The model under review builds one solid part; all positions refer to its coordinate system, in mm. Face numbers are marked on the shaded views. A direction names the side the tool comes from. Give positions to 0.01 mm unless a question says otherwise; leave off trailing zeros. Write each loop counter-clockwise with the first axis right and the second up, starting at its lowest first coordinate (ties: lowest second). Pieces come first, ordered by that corner, then holes.
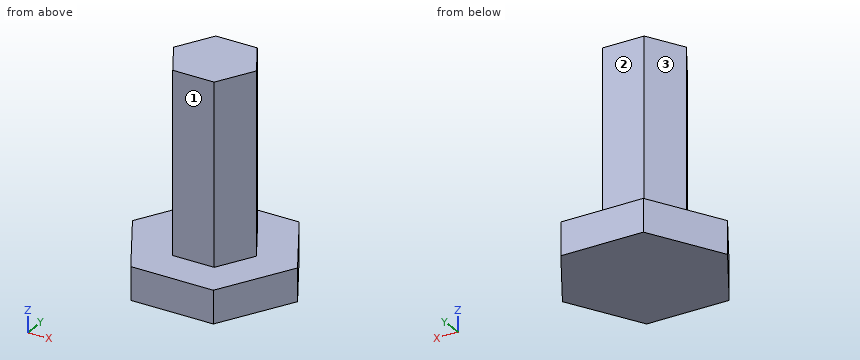
from build123d import *

# Parameters (mm, degrees)
BOSS_EXTRUDE1_DEPTH = 10
BOSS_EXTRUDE2_DEPTH = 2
MOVE_FACE1_BY       = 0.15
MOVE_FACE1_2_BY     = 0.15
MOVE_FACE1_3_BY     = 0.15
MOVE_FACE1_4_BY     = 0.15
MOVE_FACE1_5_BY     = 0.15
MOVE_FACE1_6_BY     = 0.15
MOVE_FACE1_7_BY     = 0.15
MOVE_FACE1_8_BY     = 0.15
MOVE_FACE1_9_BY     = 0.15
MOVE_FACE1_10_BY    = 0.15
MOVE_FACE1_11_BY    = 0.15
MOVE_FACE1_12_BY    = 0.15
MOVE_FACE1_13_BY    = 0.15


with BuildPart() as part:
    # Sketch1 → Boss-Extrude1 (new body)
    with BuildSketch(Plane.XY):
        Polygon((-2.5, 0), (-1.25, -2.165063509), (1.25, -2.165063509), (2.5, 0), (1.25, 2.165063509), (-1.25, 2.165063509), align=None)
    extrude(amount=BOSS_EXTRUDE1_DEPTH)

    # Sketch1_3 → Boss-Extrude2 (add)
    # profile 1 of 2: a face of its own
    with BuildSketch(Plane.XY):
        Polygon((-4.809401077, 0), (-2.404700538, -4.165063509), (2.404700538, -4.165063509), (4.809401077, 0), (2.404700538, 4.165063509), (-2.404700538, 4.165063509), align=None)
        Polygon((-1.25, -2.165063509), (1.25, -2.165063509), (2.5, 0), (1.25, 2.165063509), (-1.25, 2.165063509), (-2.5, 0), align=None, mode=Mode.SUBTRACT)
    # profile 2 of 2: a face of its own
    with BuildSketch(Plane.XY):
        Polygon((-2.5, 0), (-1.25, -2.165063509), (1.25, -2.165063509), (2.5, 0), (1.25, 2.165063509), (-1.25, 2.165063509), align=None)
    extrude(amount=-BOSS_EXTRUDE2_DEPTH)

    # Move Face1: a face moved inward by 0.15
    extrude(part.faces().sort_by_distance((0, -3.332050808, 0))[0], amount=MOVE_FACE1_BY, dir=(0, 0, -1), mode=Mode.SUBTRACT)

    # Move Face1 2: a face moved inward by 0.15
    extrude(part.faces().sort_by_distance((0, 4.165063509, -1))[0], amount=MOVE_FACE1_2_BY, dir=(0, -1, 0), mode=Mode.SUBTRACT)

    # Move Face1 3: a face moved inward by 0.15
    extrude(part.faces().sort_by_distance((3.607050808, 2.082531755, -1))[0], amount=MOVE_FACE1_3_BY, dir=(-0.866025404, -0.5, 0), mode=Mode.SUBTRACT)

    # Move Face1 4: a face moved inward by 0.15
    extrude(part.faces().sort_by_distance((3.607050808, -2.082531755, -1))[0], amount=MOVE_FACE1_4_BY, dir=(-0.866025404, 0.5, 0), mode=Mode.SUBTRACT)

    # Move Face1 5: a face moved inward by 0.15
    extrude(part.faces().sort_by_distance((0, -4.165063509, -1))[0], amount=MOVE_FACE1_5_BY, dir=(0, 1, 0), mode=Mode.SUBTRACT)

    # Move Face1 6: a face moved inward by 0.15
    extrude(part.faces().sort_by_distance((-3.607050808, 2.082531755, -1))[0], amount=MOVE_FACE1_6_BY, dir=(0.866025404, -0.5, 0), mode=Mode.SUBTRACT)

    # Move Face1 7: a face moved inward by 0.15
    extrude(part.faces().sort_by_distance((-3.607050808, -2.082531755, -1))[0], amount=MOVE_FACE1_7_BY, dir=(0.866025404, 0.5, 0), mode=Mode.SUBTRACT)

    # Move Face1 8: a face moved inward by 0.15
    extrude(part.faces().sort_by_distance((1.875, 1.082531755, 5))[0], amount=MOVE_FACE1_8_BY, dir=(-0.866025404, -0.5, 0), mode=Mode.SUBTRACT)

    # Move Face1 9: a face moved inward by 0.15
    extrude(part.faces().sort_by_distance((0, 2.165063509, 5))[0], amount=MOVE_FACE1_9_BY, dir=(0, -1, 0), mode=Mode.SUBTRACT)

    # Move Face1 10: a face moved inward by 0.15
    extrude(part.faces().sort_by_distance((-1.875, 1.082531755, 5))[0], amount=MOVE_FACE1_10_BY, dir=(0.866025404, -0.5, 0), mode=Mode.SUBTRACT)

    # Move Face1 11: a face moved inward by 0.15
    extrude(part.faces().sort_by_distance((-1.875, -1.082531755, 5))[0], amount=MOVE_FACE1_11_BY, dir=(0.866025404, 0.5, 0), mode=Mode.SUBTRACT)

    # Move Face1 12: a face moved inward by 0.15
    extrude(part.faces().sort_by_distance((0, -2.165063509, 5))[0], amount=MOVE_FACE1_12_BY, dir=(0, 1, 0), mode=Mode.SUBTRACT)

    # Move Face1 13: a face moved inward by 0.15
    extrude(part.faces().sort_by_distance((1.875, -1.082531755, 5))[0], amount=MOVE_FACE1_13_BY, dir=(-0.866025404, 0.5, 0), mode=Mode.SUBTRACT)


solid = part.part
1) Consider section D-D, the plane z = -1.25. Give the boundary of the cut face in (x, y), then the cut area to 3 significant figures.
2) Insertion check: pin 1 (0.7 mm diameter, centred on x = 0.5, z = 5.5, fed in from +Y); pin 2 (2 mm diameter, centred on y = -2.5, z = 5, fed in from +X); pin 3 (1.2 mm diameter, centred on x = 0, z = 3, fed in from -Y). Each pin has a flat end and moves straight along its axis. Give the tip position at first contact, or say it passes through.
3) Consider section B-B, the plane z = 1. Give the boundary of the cut face in (x, y).
4) To check wall thickness, follow probe 1 along Z at (x, y) = (-1.5, -1.75); probe 2 along Y at (x, z) = (0, 7.5); probe 3 along X at (y, z) = (1.75, 5.5). State the ranges of each line that lie inside material, in increasing order.
5) Consider section A-A, the plane x = 0.75. Give the boundary of the cut face in (y, z).
6) Tool access review of the marked faces 1, 2 and 3: name each direction out of +Z, -Z, +X, -X, +Y, -Y from which nothing blocks a thin tool from reaching the whole face with its end or side.
7) Consider section C-C, the plane y = -0.25. Give the boundary of the cut face in (x, z), then the cut area to 3 significant figures.
Answer block:
1. outline: (-4.64, 0) - (-2.32, -4.02) - (2.32, -4.02) - (4.64, 0) - (2.32, 4.02) - (-2.32, 4.02) - close
1. area: 55.8 mm2
2. pin 1: stops at y = 2.02
2. pin 2: stops at x = 1.46
2. pin 3: stops at y = -2.02
3. outline: (-2.33, 0) - (-1.16, -2.02) - (1.16, -2.02) - (2.33, 0) - (1.16, 2.02) - (-1.16, 2.02) - close
4. probe 1: z = -2 to -0.15
4. probe 2: y = -2.02 to 2.02
4. probe 3: x = -1.32 to 1.32
5. outline: (-4.02, -2) - (4.02, -2) - (4.02, -0.15) - (2.02, -0.15) - (2.02, 10) - (-2.02, 10) - (-2.02, -0.15) - (-4.02, -0.15) - close
6. face 1: +Z, +X, -X, -Y
6. face 2: +Z, +X, -X, +Y
6. face 3: +Z, -X, +Y
7. outline: (-4.49, -2) - (4.49, -2) - (4.49, -0.15) - (2.18, -0.15) - (2.18, 10) - (-2.18, 10) - (-2.18, -0.15) - (-4.49, -0.15) - close
7. area: 60.9 mm2
